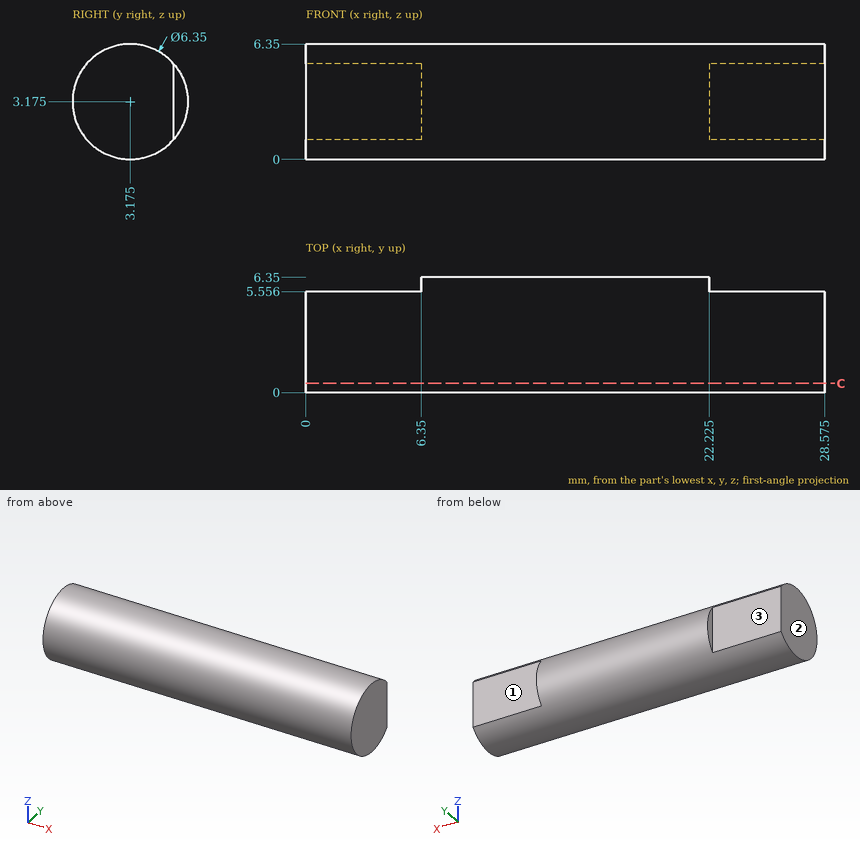
Input: dimensioned drawing with shaded views. Units: mm. Origin: part minimum x, y, z. A direction names the side the tool comes from. Give positions to 0.01 mm unless a question says otherwise; leave off trailing zeros. Write each loop counter-clockwise with the first axis right and the second up, starting at its lowest first coordinate (ties: lowest second). Pieces come first, ordered by that corner, then holes.
Q1. Set-up query: the marked faces 1, 2 and 3. Return all of +Z, -Z, +X, -X, +Y, -Y with unobstructed straight access to the full face (end or side cutting, diameter ignored); none if empty.
Q2. First-contact query: P1, Ø1.3, axis at x = 2.5, z = 4, coming from the +Y side. Flat tip, straight axial feed; report the tip coordinate or a pass-through.
Q3. Section C-C, the plane y = 0.5. Output: boundary loops of the cut face in (x, z) (1 decimal).
Q4. Material intervals for probe 1 along Z at (x, y) = (8.5, 3.25); probe 2 along Y at (x, z) = (20.25, 2) (1 decimal); probe 3 along Y at (x, z) = (13.5, 1.5), sorted ascending.
Filled in:
1. face 1: +Z, -Z, +X, +Y
1. face 2: +Z, -Z, -X, +Y, -Y
1. face 3: +Z, -Z, -X, +Y
2. P1: stops at y = 5.56
3. outline: (0, 1.5) - (28.6, 1.5) - (28.6, 4.9) - (0, 4.9) - close
4. probe 1: z = 0 to 6.35
4. probe 2: y = 0.2 to 6.1
4. probe 3: y = 0.48 to 5.87
